Read the model definition and answer for the solid it produces. Units are mm, in the model's axes. A direction names the side the tool comes from. Coordinates: 2 decimals unless noted, no trailing zeros. Order: outer loops, then holes, each group sorted by start corner. A loop starts at its lowest first (then second) coordinate and runs counter-clockwise, first axis right, second up. Notation, with made-up numbers: (59.5, 58.5) - (68.5, 58.5) arc R33 cw to (68.5, 94.5) - close; hole circle Ø10 at (12.5, 22.5). An arc over 180 degrees is marked (long way). Write item = value, one per line.
from build123d import *

# Parameters (mm, degrees)
F0_R     = 11.2
F1_DEPTH = 25


with BuildPart() as f1:
    # F0 (on Top) → F1 (new body)
    with BuildSketch(Plane.XY):
        with BuildLine():
            ThreePointArc((3.831396, 10.524277), (9.174738, 6.42372), (11.2, 0))
            ThreePointArc((11.2, 0), (7.919596, -7.919596), (0, -11.2))
            Line((0, -11.2), (1.961414, -18.765441))
            Line((1.961414, -18.765441), (11.275878, -18.765441))
            ThreePointArc((11.275878, -18.765441), (34.854913, -19.940638), (21.662812, -0.362067))
            Line((21.662812, -0.362067), (21.662812, 6.24599))
            Line((21.662812, 6.24599), (15.962205, 7.635998))
            Line((15.962205, 7.635998), (15.147737, 13.595152))
            Line((15.147737, 13.595152), (12.678516, 16.088038))
            Line((12.678516, 16.088038), (11.0789, 17.702983))
            Line((11.0789, 17.702983), (3.831396, 10.524277))
        make_face()
        with Locations((23.359479, -13.452572)):
            Circle(F0_R, mode=Mode.SUBTRACT)
        with BuildLine():
            ThreePointArc((-5.568315, 9.717709), (-0.957528, 11.158994), (3.831396, 10.524277))
            Line((3.831396, 10.524277), (11.0789, 17.702983))
            Line((11.0789, 17.702983), (10.209294, 18.580924))
            ThreePointArc((10.209294, 18.580924), (1.201666, 40.09333), (-11.557174, 20.570703))
            Line((-11.557174, 20.570703), (-5.568315, 9.717709))
        make_face()
        with Locations((0, 26.948141)):
            Circle(F0_R, mode=Mode.SUBTRACT)
        with BuildLine():
            Line((1.961414, -18.765441), (0, -11.2))
            ThreePointArc((0, -11.2), (-10.823085, -2.881116), (-5.568315, 9.717709))
            Line((-5.568315, 9.717709), (-11.557174, 20.570703))
            Line((-11.557174, 20.570703), (-17.183078, 16.615154))
            Line((-17.183078, 16.615154), (-15.250741, 9.161863))
            Line((-15.250741, 9.161863), (-20.906688, 7.635998))
            Line((-20.906688, 7.635998), (-18.528908, -1.177754))
            ThreePointArc((-18.528908, -1.177754), (-35.495636, -18.552516), (-11.211755, -18.765441))
            Line((-11.211755, -18.765441), (1.961414, -18.765441))
        make_face()
        with Locations((-23.308304, -13.482118)):
            Circle(F0_R, mode=Mode.SUBTRACT)
    extrude(amount=F1_DEPTH)


solid = f1.part
1) The part is cut by section A-A (x = 31.5). Determine the outline of the cut face in (y, z).
Returned:
outline = (-23.84, 0) - (-21.14, 0) - (-21.14, 25) - (-23.84, 25) - close; (-5.76, 0) - (-3.06, 0) - (-3.06, 25) - (-5.76, 25) - close
2) Straight lines are drawn through the part: line 1 along X through (y, z) = (-22.5, 6.25); line 2 along X through (y, z) = (-21.5, 22.25); line 3 along Y through (x, z) = (-6, 19.5). For each, find the intervals that lie inside material, in ascending order. Write a range as from..to.
Returned:
line_1 = -32.95..-29.95, -16.67..-13.67, 13.75..16.76, 29.96..32.97
line_2 = -33.79..-31.13, -15.49..-12.82, 12.9..15.57, 31.15..33.82
line_3 = -18.77..-9.46, 9.46..17.49, 36.41..38.71
3) The part is cut by section D-D (y = -16). Determine the outline of the cut face in (x, z) (3 decimals).
Returned:
outline = (-36.266, 0) - (-34.222, 0) - (-34.222, 25) - (-36.266, 25) - close; (-12.395, 0) - (12.453, 0) - (12.453, 25) - (-12.395, 25) - close; (34.266, 0) - (36.311, 0) - (36.311, 25) - (34.266, 25) - close
4) Flat-ended cylindrical pins translate along their axes: pin 1 Ø12 at (x, y) = (-11, 5) entering from -Z; pin 2 Ø10 at (x, z) = (-16, 12.5) entering from +Y; pin 3 Ø7.5 at (y, z) = (1.5, 12.5) entering from +X; pin 4 Ø1 at (x, z) = (-26, 21) entering from -Y. Find the tip coordinate at first contact, or state that the pin passes through.
Returned:
pin_1 = 0
pin_2 = 34.24
pin_3 = 30.34
pin_4 = -26.5
5) The part is cut by section C-C (x = 1.5). Determine the outline of the cut face in (y, z), and give its area (3 significant figures).
Returned:
outline = (-18.77, 0) - (-11.1, 0) - (-11.1, 25) - (-18.77, 25) - close; (11.1, 0) - (15.85, 0) - (15.85, 25) - (11.1, 25) - close; (38.05, 0) - (40.06, 0) - (40.06, 25) - (38.05, 25) - close
area = 361 mm^2
6) Determine the mould class of faces 1 (the face through (21.663, 3, 12)), 2 (the face through (-19.734, 3.291, 12.325)), 3 (the face through (18.85, 6.93, 12.32)) for opening direction Y: pulls with the +Y half, pulls with the -Y half, needs draft (parallel to the pull), parting line crosses it, or undercut.
Returned:
face_1 = needs draft
face_2 = undercut
face_3 = pulls with the +Y half
7) The part is cut by section B-B (y = 3.5). Determine the outline of the cut face in (x, z).
Returned:
outline = (-19.79, 0) - (-10.64, 0) - (-10.64, 25) - (-19.79, 25) - close; (10.64, 0) - (21.66, 0) - (21.66, 25) - (10.64, 25) - close
8) For faces 4 (the face through (-14.33, 18.62, 12.32)), 5 (the face through (0, -18.765, 12)), 6 (the face through (1.6, 40.05, 12.32)), determine the directions among +Z, -Z, +X, -X, +Y, -Y from which every point of the face is accessible in a straight line to the end or side of a thin tool.
Returned:
face_4 = +Z, -Z, -X
face_5 = +Z, -Z, -Y
face_6 = +Z, -Z
